Geometry check sheet. Reference: the model listing, model coordinates, mm. Face numbers are marked on the shaded views. Round coordinates to 2 decimals unless told otherwise and drop trailing zeros. Write each loop counter-clockwise with the first axis right and the second up, starting at its lowest first coordinate (ties: lowest second). Pieces come first, ordered by that corner, then holes.
from build123d import *

# Parameters (mm, degrees)
CROQUIS1_R              = 11.5
SALIENTE_EXTRUIR1_DEPTH = 19.5
SALIENTE_EXTRUIR2_START = 2
CROQUIS2_R              = 1.625
SALIENTE_EXTRUIR2_DEPTH = 2


with BuildPart() as part:
    # Croquis1 → Saliente-Extruir1 (new body)
    with BuildSketch(Plane.XY):
        with BuildLine():
            Line((0.964194139, 12.964194139), (0, 12))
            Line((0, 12), (-0.964194139, 12.964194139))
            ThreePointArc((-0.964194139, 12.964194139), (-9.192388155, 9.192388155), (-12.964194139, 0.964194139))
            Line((-12.964194139, 0.964194139), (-12, 0))
            Line((-12, 0), (-12.964194139, -0.964194139))
            ThreePointArc((-12.964194139, -0.964194139), (-9.192388155, -9.192388155), (-0.964194139, -12.964194139))
            Line((-0.964194139, -12.964194139), (0, -12))
            Line((0, -12), (0.964194139, -12.964194139))
            ThreePointArc((0.964194139, -12.964194139), (9.192388155, -9.192388155), (12.964194139, -0.964194139))
            Line((12.964194139, -0.964194139), (12, 0))
            Line((12, 0), (12.964194139, 0.964194139))
            ThreePointArc((12.964194139, 0.964194139), (9.192388155, 9.192388155), (0.964194139, 12.964194139))
        make_face()
        Circle(CROQUIS1_R, mode=Mode.SUBTRACT)
    extrude(amount=-SALIENTE_EXTRUIR1_DEPTH)

    # Croquis2 → Saliente-Extruir2 (add)
    with BuildSketch(Plane.XY.offset(SALIENTE_EXTRUIR2_START)):
        with BuildLine():
            Line((-12.964194139, -0.964194139), (-12, 0))
            Line((-12, 0), (-12.964194139, 0.964194139))
            ThreePointArc((-12.964194139, 0.964194139), (-9.192388155, 9.192388155), (-0.964194139, 12.964194139))
            Line((-0.964194139, 12.964194139), (0, 12))
            Line((0, 12), (0.964194139, 12.964194139))
            ThreePointArc((0.964194139, 12.964194139), (9.192388155, 9.192388155), (12.964194139, 0.964194139))
            Line((12.964194139, 0.964194139), (12, 0))
            Line((12, 0), (12.964194139, -0.964194139))
            ThreePointArc((12.964194139, -0.964194139), (9.192388155, -9.192388155), (0.964194139, -12.964194139))
            Line((0.964194139, -12.964194139), (0, -12))
            Line((0, -12), (-0.964194139, -12.964194139))
            ThreePointArc((-0.964194139, -12.964194139), (-9.192388155, -9.192388155), (-12.964194139, -0.964194139))
        make_face()
        Circle(CROQUIS2_R, mode=Mode.SUBTRACT)
        with Locations((6, 0)):
            Circle(CROQUIS2_R, mode=Mode.SUBTRACT)
        with Locations((-6, 0)):
            Circle(CROQUIS2_R, mode=Mode.SUBTRACT)
        with Locations((0, 6)):
            Circle(CROQUIS2_R, mode=Mode.SUBTRACT)
        with Locations((0, -6)):
            Circle(CROQUIS2_R, mode=Mode.SUBTRACT)
    extrude(amount=-SALIENTE_EXTRUIR2_DEPTH)


solid = part.part
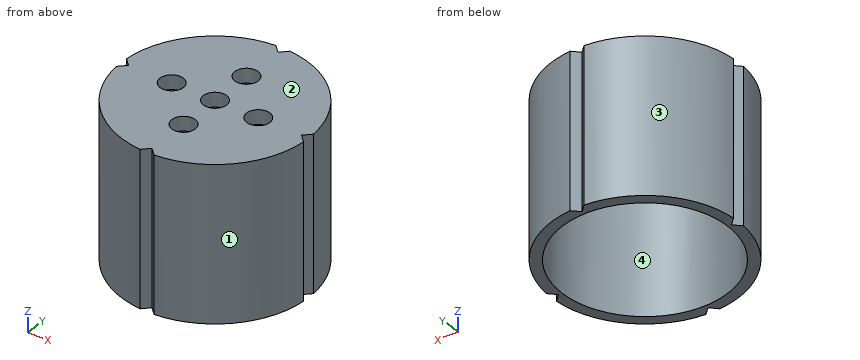
1. Section check B-B (y = 6). Record the cut outline in (x, z) (3 decimals), plus the area to 3 significant figures.
2. Section check A-A (z = -6.25). Record the cut outline in (x, y), plus the area to 3 significant figures.
3. Section check D-D (x = 3). Record the cut outline in (y, z).
4. Scan lines: line 1 along Y through (x, z) = (9, -9); line 2 along Y through (x, z) = (4.5, -11.75); line 3 along Z through (x, y) = (-3.25, 0.25). Record each from-to range of solid material in increasing order.
5. Section check C-C (x = -5.75). Record the cut outline in (y, z).
6. Depth check by flat-ended pin: pin 1 Ø5 at (x, y) = (0, 6) entering from +Z; pin 2 Ø8 at (y, z) = (-8, -6) entering from -X; pin 3 Ø4 at (x, z) = (8.5, -4) entering from -Y; pin 4 Ø2.5 at (x, y) = (0, -6) entering from -Z. Enter the tip coordinate at first touch or a pass-through.
7. Release check for a two-part mould opening along Y. For the marked faces 1, 2, 3 and 4 record: +Y half, -Y half, draft (parallel to the pull), parting line (faces both ways), or undercut.
Results below:
1. outline: (-11.533, -19.5) - (-9.811, -19.5) - (-9.811, 0) - (-1.625, 0) - (-1.625, 2) - (-11.533, 2) - close; (1.625, 0) - (9.811, 0) - (9.811, -19.5) - (11.533, -19.5) - (11.533, 2) - (1.625, 2) - close
1. area: 107 mm2
2. outline: (-12.96, -0.96) arc R13 ccw to (-0.96, -12.96) - (0, -12) - (0.96, -12.96) arc R13 ccw to (12.96, -0.96) - (12, 0) - (12.96, 0.96) arc R13 ccw to (0.96, 12.96) - (0, 12) - (-0.96, 12.96) arc R13 ccw to (-12.96, 0.96) - (-12, 0) - close; hole circle Ø23 at (0, 0)
2. area: 112 mm2
3. outline: (-12.65, -19.5) - (-11.1, -19.5) - (-11.1, 0) - (11.1, 0) - (11.1, -19.5) - (12.65, -19.5) - (12.65, 2) - (-12.65, 2) - close
4. line 1: y = -9.38 to -7.16, 7.16 to 9.38
4. line 2: y = -12.2 to -10.58, 10.58 to 12.2
4. line 3: z = 0 to 2
5. outline: (-11.66, -19.5) - (-9.96, -19.5) - (-9.96, 0) - (-1.61, 0) - (-1.61, 2) - (-11.66, 2) - close; (1.61, 0) - (9.96, 0) - (9.96, -19.5) - (11.66, -19.5) - (11.66, 2) - (1.61, 2) - close
6. pin 1: stops at z = 2
6. pin 2: stops at x = -12.37
6. pin 3: stops at y = -11.26
6. pin 4: passes through
7. face 1: -Y half
7. face 2: draft
7. face 3: +Y half
7. face 4: undercut
